from build123d import *

# Parameters (mm, degrees)
BOSS_EXTRUDE1_DEPTH = 2
BOSS_EXTRUDE2_START = 3.5
SKETCH2_R           = 1.6
BOSS_EXTRUDE2_DEPTH = 3.5


with BuildPart() as part:
    # Sketch1 → Boss-Extrude1 (new body)
    with BuildSketch(Plane(origin=(0, 0, 0), x_dir=(1, 0, 0), z_dir=(0, 1, 0))):
        with BuildLine():
            Line((-3.45, 2.4), (3.45, 2.4))
            ThreePointArc((3.45, 2.4), (5.85, 0), (3.45, -2.4))
            Line((3.45, -2.4), (-3.45, -2.4))
            ThreePointArc((-3.45, -2.4), (-5.85, 0), (-3.45, 2.4))
        make_face()
        with BuildLine():
            Line((-4.05, 1.15), (4.05, 1.15))
            ThreePointArc((4.05, 1.15), (5.2, 0), (4.05, -1.15))
            Line((4.05, -1.15), (-4.05, -1.15))
            ThreePointArc((-4.05, -1.15), (-5.2, 0), (-4.05, 1.15))
        make_face(mode=Mode.SUBTRACT)
    extrude(amount=BOSS_EXTRUDE1_DEPTH)

    # Sketch2 → Boss-Extrude2 (add)
    with BuildSketch(Plane.XZ.offset(BOSS_EXTRUDE2_START)):
        with BuildLine():
            Line((-8.05, 5.95), (8.05, 5.95))
            ThreePointArc((8.05, 5.95), (14, 0), (8.05, -5.95))
            Line((8.05, -5.95), (-8.05, -5.95))
            ThreePointArc((-8.05, -5.95), (-14, 0), (-8.05, 5.95))
        make_face()
        with Locations(Location((-10, 0, 0), (0, 0, 270))):
            Circle(SKETCH2_R, mode=Mode.SUBTRACT)
        with Locations(Location((10, 0, 0), (0, 0, 270))):
            Circle(SKETCH2_R, mode=Mode.SUBTRACT)
        with BuildLine():
            Line((4.05, -1.15), (-4.05, -1.15))
            ThreePointArc((-4.05, -1.15), (-5.2, 0), (-4.05, 1.15))
            Line((-4.05, 1.15), (4.05, 1.15))
            ThreePointArc((4.05, 1.15), (5.2, 0), (4.05, -1.15))
        make_face(mode=Mode.SUBTRACT)
    extrude(amount=-BOSS_EXTRUDE2_DEPTH)


solid = part.part
Source: CAD feature listing. Evaluate the final solid. Frame: model axes, mm. A direction names the side the tool comes from. Round coordinates to 2 decimals unless told otherwise and drop trailing zeros. Loops run counter-clockwise (first coordinate to the right, second up) from the corner with the lowest first, then second, coordinate; pieces in that order, holes last.
Q1. Ray query, line 1 (X direction, y = -2.2, z = 0); line 2 (Y direction, x = 9.75, z = -2.25); line 3 (Z direction, x = 10.75, y = -0.95). Return the intervals inside material, ascending.
Q2. First-contact query: P1, Ø0.6, axis at x = -1, y = 0.5, coming from the +Z side; P2, Ø3.5, axis at x = -10, z = 0, coming from the +Y side; P3, Ø1, axis at x = 9.5, y = -3, coming from the +Z side. Flat tips, straight axial feed; report the tip coordinate or a pass-through.
Q3. Section A-A, the plane z = 0. Return loops of the section in (x, y), plus the area to 3 significant figures.
Q4. Section D-D, the plane y = -2.25. Return loops of the section in (x, z).
Q5. Mould query, pull axis Z, two halves, no side actions, for faces 1 (the face through (5.85, 0.99, -0.05)), 2 (the face through (0.2, -3.5, 1.4)), 3 (the face through (0, -1, 1.15)). Classes: pulls with the +Z half, pulls with the -Z half, needs draft (parallel to the pull), parting line crosses it, or undercut.
Q6. Section C-C, the plane x = -2. Return loops of the section in (y, z), plus the area to 3 significant figures.
Q7. Section B-B, the plane y = 1.35. Return loops of the section in (x, z).
Q8. Access query for faces 4 (the face through (-5.85, 0.99, 0.05)), 5 (the face through (0, -1, -1.15)), 6 (the face through (0, 1, -2.4)), 7 (the face through (0, 1, 2.4)). Directions: +Z, -Z, +X, -X, +Y, -Y. A direction counts if a zero-diameter tool reaches every point of the face in a straight line with its end or side. Return the directions, or none.
Solutions:
1. line 1: x = -14 to -11.6, -8.4 to -5.2, 5.2 to 8.4, 11.6 to 14
1. line 2: y = -3.5 to 0
1. line 3: z = -5.3 to -1.41, 1.41 to 5.3
2. P1: stops at z = 2.4
2. P2: stops at y = 0
2. P3: stops at z = 5.87
3. outline: (-14, -3.5) - (-11.6, -3.5) - (-11.6, 0) - (-14, 0) - close; (-8.4, -3.5) - (-5.2, -3.5) - (-5.2, 2) - (-5.85, 2) - (-5.85, 0) - (-8.4, 0) - close; (5.2, -3.5) - (8.4, -3.5) - (8.4, 0) - (5.85, 0) - (5.85, 2) - (5.2, 2) - close; (11.6, -3.5) - (14, -3.5) - (14, 0) - (11.6, 0) - close
3. area: 41.8 mm2
4. outline: (-8.05, -5.95) - (8.05, -5.95) arc R5.95 ccw to (8.05, 5.95) - (-8.05, 5.95) arc R5.95 ccw to start; hole circle Ø3.2 at (-10, 0); hole (-4.05, -1.15) - (4.05, -1.15) arc R1.15 ccw to (4.05, 1.15) - (-4.05, 1.15) arc R1.15 ccw to start; hole circle Ø3.2 at (10, 0)
5. face 1: parting line crosses it
5. face 2: needs draft
5. face 3: undercut
6. outline: (-3.5, -5.95) - (0, -5.95) - (0, -2.4) - (2, -2.4) - (2, -1.15) - (-3.5, -1.15) - close; (-3.5, 1.15) - (2, 1.15) - (2, 2.4) - (0, 2.4) - (0, 5.95) - (-3.5, 5.95) - close
6. area: 38.6 mm2
7. outline: (-3.45, -2.4) - (3.45, -2.4) arc R2.4 ccw to (3.45, 2.4) - (-3.45, 2.4) arc R2.4 ccw to start; hole (-4.05, -1.15) - (4.05, -1.15) arc R1.15 ccw to (4.05, 1.15) - (-4.05, 1.15) arc R1.15 ccw to start
8. face 4: -X, +Y
8. face 5: +Y, -Y
8. face 6: -Z, +X, -X, +Y
8. face 7: +Z, +X, -X, +Y
